```python
from build123d import *

# Parameters (mm, degrees)
SKETCH1_R           = 10.31875
BOSS_EXTRUDE1_DEPTH = 1.5875
SKETCH2_R           = 8.73125
BOSS_EXTRUDE2_DEPTH = 6.35
SKETCH3_R           = 6.35
BOSS_EXTRUDE3_DEPTH = 1.5875
SKETCH4_R           = 4.7625
SKETCH4_R_2         = 3.96875
CUT_EXTRUDE1_DEPTH  = 0.254
CUT_EXTRUDE2_START  = -0.254
SKETCH5_R           = 9.23925
SKETCH5_R_2         = 8.73125
CUT_EXTRUDE2_DEPTH  = 0.254
SKETCH6_R           = 3.175
CUT_EXTRUDE3_DEPTH  = 18.426383105
CHAMFER1_SIZE       = 0.254


with BuildPart() as part:
    # Sketch1 → Boss-Extrude1 (new body)
    with BuildSketch(Plane.XY):
        Circle(SKETCH1_R)
    extrude(amount=BOSS_EXTRUDE1_DEPTH)

    # Sketch2 → Boss-Extrude2 (add)
    with BuildSketch(Plane.XY.offset(1.5875)):
        Circle(SKETCH2_R)
    extrude(amount=BOSS_EXTRUDE2_DEPTH)

    # Sketch3 → Boss-Extrude3 (add)
    with BuildSketch(Plane(origin=(0, 0, 0), x_dir=(-1, 0, 0), z_dir=(0, 0, -1))):
        with Locations(Location((0, 0, 0), (0, 0, 180))):
            Circle(SKETCH3_R)
    extrude(amount=BOSS_EXTRUDE3_DEPTH)

    # Sketch4 → Cut-Extrude1 (cut)
    with BuildSketch(Plane(origin=(0, 0, -1.5875), x_dir=(-1, 0, 0), z_dir=(0, 0, -1))):
        Circle(SKETCH4_R)
        Circle(SKETCH4_R_2, mode=Mode.SUBTRACT)
    extrude(amount=-CUT_EXTRUDE1_DEPTH, mode=Mode.SUBTRACT)

    # Sketch5 → Cut-Extrude2 (cut)
    with BuildSketch(Plane.XY.offset(1.5875).offset(CUT_EXTRUDE2_START)):
        Circle(SKETCH5_R)
        Circle(SKETCH5_R_2, mode=Mode.SUBTRACT)
    extrude(amount=CUT_EXTRUDE2_DEPTH, mode=Mode.SUBTRACT)

    # Sketch6 → Cut-Extrude3 (cut, through all)
    with BuildSketch(Plane.XY.offset(7.9375)):
        Circle(SKETCH6_R)
    extrude(amount=-CUT_EXTRUDE3_DEPTH, mode=Mode.SUBTRACT)

    # Chamfer1
    chamfer1_edges = [part.edges().sort_by_distance(p)[0] for p in [
        (3.96875, 0, -1.5875),
        (-3.175, 0, -1.5875),
        (-3.175, 0, 7.9375),
    ]]
    chamfer(chamfer1_edges, length=CHAMFER1_SIZE - 0.0001)  # a hair under: the kernel refuses the full size


solid = part.part
```
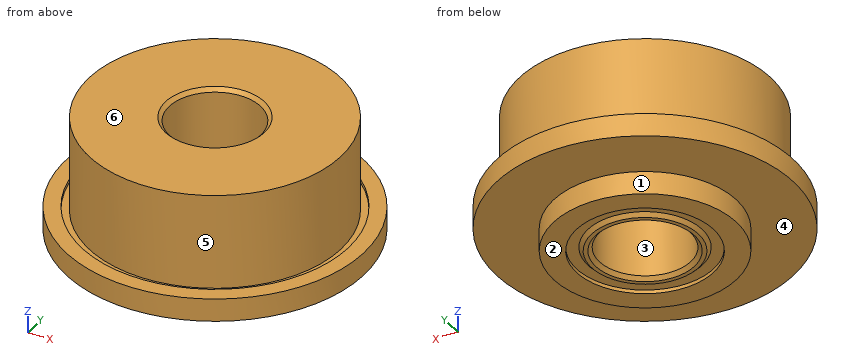
Part model, mm, in its own coordinate system. Face numbers are marked on the shaded views. A direction names the side the tool comes from. Round coordinates to 2 decimals unless told otherwise and drop trailing zeros. Loops run counter-clockwise (first coordinate to the right, second up) from the corner with the lowest first, then second, coordinate; pieces in that order, holes last. Notation, with made-up numbers: (-5, 56) -> (10, 56) arc R16 cw to (10, 83) -> close; hole circle Ø8 at (-20.75, 60). An arc over 180 degrees is marked (long way). Use one line per item in the form item = value. Start each with the question number.
Item 1: Drill centre lines: line 1 along Y through (x, z) = (0, 1.5) (3 decimals); line 2 along Y through (x, z) = (4, 1.5); line 3 along Y through (x, z) = (0, -1.45). Where is each one in solid material? Low to high.
Item 2: Tool access for the marked faces 4, 5 and 6: list every direction of +Z, -Z, +X, -X, +Y, -Y with a clear straight run to the whole face (end or side of a thin tool).
Item 3: Drop flat-ended pins along their axis: pin 1 Ø1.5 at (y, z) = (-7, 3) entering from +X; pin 2 Ø4 at (y, z) = (5, 4) entering from -X; pin 3 Ø5 at (y, z) = (4, 3.5) entering from +X. Give the stop position or say it passes through.
Item 4: Band-saw the part on C-C (x = -7.75). List the corners of the cut face in (y, z), plus the area to 3 significant figures.
Item 5: Band-saw the part on B-B (z = -0.25). List the corners of the cut face in (x, y) (3 decimals).
Item 6: Two-plate mould, pull along X, no slides. Class the marked faces 1, 2 and 3: released by +X, released by -X, zero draft, split by the parting line, or undercut.
Data:
q1.line_1 = -10.319 to -9.239, -8.731 to -3.175, 3.175 to 8.731, 9.239 to 10.319
q1.line_2 = -9.51 to -8.33, -7.76 to 7.76, 8.33 to 9.51
q1.line_3 = -6.35 to -4.76, -3.85 to -3.29, 3.29 to 3.85, 4.76 to 6.35
q2.face_4 = -Z
q2.face_5 = +Z
q2.face_6 = +Z, +X, -X, +Y, -Y
q3.pin_1 = 6.1
q3.pin_2 = -8.2
q3.pin_3 = 10.04
q4.outline = (-6.81, 0) -> (6.81, 0) -> (6.81, 1.59) -> (5.03, 1.59) -> (5.03, 1.33) -> (4.02, 1.33) -> (4.02, 7.94) -> (-4.02, 7.94) -> (-4.02, 1.33) -> (-5.03, 1.33) -> (-5.03, 1.59) -> (-6.81, 1.59) -> close
q4.area = 72.2 mm^2
q5.outline = circle Ø12.7 at (0, 0); hole circle Ø6.35 at (0, 0)
q6.face_1 = split by the parting line
q6.face_2 = zero draft
q6.face_3 = undercut
